Autodesk Fusion 360 part; units mm, degrees
sketch "Skizze1" plane through (0, 0, 0) normal (0, 1, 0) x (1, 0, 0)
  line L0 (0, 0) -> (827, 0)
  line L1 (827, 0) -> (827, -195)
  line L2 (827, -195) -> (0, -195)
  line L3 (0, -195) -> (0, 0)
  line L4 (0, -195) -> (128, -195)
  line L5 (128, -195) -> (128, -70)
  line L6 (128, -70) -> (228, -70)
  line L7 (228, -70) -> (228, 0)
  line L8 (228, 0) -> (128, 0)
  line L9 (128, 0) -> (128, -70)
  dimension "d1" = 827
  dimension "d2" = 195
  dimension "d3" = 128
  dimension "d4" = 125
  dimension "d5" = 100
  dimension "d6" = 70
extrude "Extrusion1" add sketch "Skizze1" along normal blind 5 contours L0 L2 L3 L4 L5 L9 | L0 L1 L2 L5 L6 L7
extrude "Extrusion2" add 2 faces at (427.6667, 1.6667, 0) (42.6667, 3.3333, 0) along direction (0, 0, -1) blind 1
sketch "Skizze2" plane through (0, 5, 0) normal (0, 1, 0) x (-1, 0, 0)
  line L0 (0, 195) -> (-827, 195)
  line L1 (-827, 195) -> (-827, -1)
  line L2 (-827, -1) -> (-228, -1)
  line L3 (-228, -1) -> (-228, 70)
  line L4 (-228, 70) -> (-128, 70)
  line L5 (-128, 70) -> (-128, -1)
  line L6 (-128, -1) -> (0, -1)
  line L7 (0, -1) -> (0, 195)
  line L8 (-128, -1) -> (-228, -1)
  line L9 (-128, -1) -> (-128, 0)
  line L10 (-128, 0) -> (-228, 0)
  line L11 (-228, -1) -> (-228, 0)
extrude "Extrusion3" add sketch "Skizze2" against normal blind 5 contours L3 L5 L8 L9 L10 L11
sketch "Skizze3" plane through (0, 5, 0) normal (0, 1, 0) x (-1, 0, 0)
  line L0 (-228, 0) -> (-228, 70)
  line L1 (-228, 70) -> (-128, 70)
  line L2 (-128, 70) -> (-128, 0)
  line L3 (-128, 0) -> (-228, 0)
  line L4 (-827, -1) -> (0, -1)
  line L5 (0, -1) -> (0, 195)
  line L6 (0, 195) -> (-827, 195)
  line L7 (-827, 195) -> (-827, -1)
  line L8 (0, 195) -> (-354, 195)
  line L9 (-354, 195) -> (-354, 178)
  line L10 (-354, 178) -> (-431.5, 178)
  line L11 (-431.5, 178) -> (-431.5, 16)
  line L12 (-431.5, 16) -> (-354, 16)
  line L13 (-354, 16) -> (-354, 178)
  dimension "d13" = 354
  dimension "d14" = 17
  dimension "d15" = 77.5
  dimension "d16" = 162
extrude "Extrusion4" cut sketch "Skizze3" against normal blind 5 contours L10 L11 L12 L13
sketch "Skizze4" plane through (0, 5, 0) normal (0, 1, 0) x (-1, 0, 0)
  line L0 (-431.5, 178) -> (-354, 178)
  line L1 (-354, 178) -> (-354, 16)
  line L2 (-354, 16) -> (-431.5, 16)
  line L3 (-228, 0) -> (-228, 70)
  line L4 (-228, 70) -> (-128, 70)
  line L5 (-128, 70) -> (-128, 0)
  line L6 (-128, 0) -> (-228, 0)
  line L7 (-827, -1) -> (0, -1)
  line L8 (0, -1) -> (0, 195)
  line L9 (0, 195) -> (-827, 195)
  line L10 (-827, 195) -> (-827, -1)
  line L11 (-827, -1) -> (-531, -1)
  line L12 (-531, -1) -> (-531, 195)
  line L13 (-531, 195) -> (-531, 33)
  line L14 (-531, 33) -> (-496, 33)
  line L15 (-496, 33) -> (-496, 3)
  line L16 (-496, 3) -> (-531, 3)
  line L17 (-531, 3) -> (-531, 33)
  line L18 (-431.5, 16) -> (-474.5, 16)
  line L19 (-474.5, 16) -> (-397, 16)
  line L20 (-397, 16) -> (-397, 178)
  line L21 (-397, 178) -> (-474.5, 178)
  line L22 (-474.5, 178) -> (-474.5, 16)
  dimension "d19" = 296
  dimension "d20" = 162
  dimension "d21" = 35
  dimension "d22" = 30
  dimension "d23" = 43
  dimension "d24" = 162
  dimension "d25" = 77.5
extrude "Extrusion5" add sketch "Skizze4" against normal blind 5 contours L0 L1 L2 L20
sketch "Skizze5" plane through (0, 5, 0) normal (0, 1, 0) x (-1, 0, 0)
extrude "Extrusion6" cut sketch "Skizze4" against normal blind 40 contours L0 L2 L18 L19 L20 L21 L22
sketch "Skizze6" plane through (0, 5, 0) normal (0, 1, 0) x (-1, 0, 0)
  line L0 (-827, -1) -> (0, -1)
  line L1 (0, -1) -> (0, 195)
  line L2 (0, 195) -> (-827, 195)
  line L3 (-827, 195) -> (-827, -1)
  line L4 (-228, 0) -> (-228, 70)
  line L5 (-228, 70) -> (-128, 70)
  line L6 (-128, 70) -> (-128, 0)
  line L7 (-128, 0) -> (-228, 0)
  line L8 (-397, 16) -> (-474.5, 16)
  line L9 (-474.5, 16) -> (-474.5, 178)
  line L10 (-474.5, 178) -> (-397, 178)
  line L11 (-397, 178) -> (-397, 16)
  line L12 (-474.5, 16) -> (-517.5, 16)
  line L13 (-827, 195) -> (-827, 31)
  line L14 (-827, 31) -> (-474.5, 31)
  line L15 (-517.5, 16) -> (-517.5, 31)
  line L16 (-517.5, 31) -> (-552.5, 31)
  line L17 (-552.5, 31) -> (-552.5, 1)
  line L18 (-552.5, 1) -> (-517.5, 1)
  line L19 (-517.5, 1) -> (-517.5, 31)
  dimension "d30" = 43
  dimension "d31" = 164
  dimension "d32" = 35
  dimension "d33" = 30
extrude "Extrusion7" cut sketch "Skizze6" against normal blind 50 contours L14 L15 L16 L17 L18 L19
extrude "Extrusion8" add 1 faces at (275.6667, 3.3333, -1) along direction (0, 0, -1) blind 41
Geometry check sheet. Reference: the model listing, model coordinates, mm. Give positions to 0.01 mm unless a question says otherwise; leave off trailing zeros. Order: outer loops, then holes, each group sorted by start corner. A loop starts at its lowest first (then second) coordinate and runs counter-clockwise, first axis right, second up.
1. Draft check along Y on faces 1 (the face through (419, 0, -1)), 2 (the face through (500, 5, 78)). Enter one of: pulls with the +Y half, pulls with the -Y half, needs draft (parallel to the pull), parting line crosses it, or undercut.
Completed:
face 1: pulls with the -Y half
face 2: pulls with the +Y half
2. Sectioned sample at C-C (y = 1.8). Record the boundary of the cut face in (x, z), then the cut area to 3 significant figures.
Completed:
outline: (0, -42) - (827, -42) - (827, 195) - (0, 195) - close; hole (128, 0) - (228, 0) - (228, 70) - (128, 70) - close; hole (397, 16) - (474.5, 16) - (474.5, 178) - (397, 178) - close; hole (517.5, 1) - (552.5, 1) - (552.5, 31) - (517.5, 31) - close
area: 175,000 mm2
3. Sectioned sample at D-D (z = 111). Record the boundary of the cut face in (x, y), then the cut area to 3 significant figures.
Completed:
outline: (0, 0) - (397, 0) - (397, 5) - (0, 5) - close; (474.5, 0) - (827, 0) - (827, 5) - (474.5, 5) - close
area: 3,750 mm2
4. Sectioned sample at A-A (z = 47). Record the boundary of the cut face in (x, y), then the cut area to 3 significant figures.
Completed:
outline: (0, 0) - (128, 0) - (128, 5) - (0, 5) - close; (228, 0) - (397, 0) - (397, 5) - (228, 5) - close; (474.5, 0) - (827, 0) - (827, 5) - (474.5, 5) - close
area: 3,250 mm2
5. Sectioned sample at B-B (x = 460.5). Record the boundary of the cut face in (y, z), then the cut area to 3 significant figures.
Completed:
outline: (0, -42) - (5, -42) - (5, 16) - (0, 16) - close; (0, 178) - (5, 178) - (5, 195) - (0, 195) - close
area: 375 mm2
6. Scan lines: line 1 (X direction, y = 3.4, z = 30); line 2 (X direction, y = 2.55, z = 46); line 3 (X direction, y = 4.85, z = 81). Record each from-to range of solid material in increasing order.
Completed:
line 1: x = 0 to 128, 228 to 397, 474.5 to 517.5, 552.5 to 827
line 2: x = 0 to 128, 228 to 397, 474.5 to 827
line 3: x = 0 to 397, 474.5 to 827
